```python
from build123d import *

# Parameters (mm, degrees)
SKETCH_1_R      = 5
EXTRUDE_1_DEPTH = 1
SKETCH_3_R      = 3
SKETCH_2_R      = 3.75


with BuildPart() as part:
    # Эскиз1 → Бобышка-Вытянуть1 (new body)
    with BuildSketch(Plane.XY):
        with BuildLine():
            Line((-57.368421028, 25.472814244), (-33.289473642, 43.781399484))
            ThreePointArc((-33.289473642, 43.781399484), (54.999999965, 0), (-33.289473642, -43.781399484))
            Line((-33.289473642, -43.781399484), (-57.368421028, -25.472814244))
            ThreePointArc((-57.368421028, -25.472814244), (-69.999999979, 0), (-57.368421028, 25.472814244))
        make_face()
        with Locations((-22.5, 38.97114317)):
            Circle(SKETCH_1_R, mode=Mode.SUBTRACT)
        with Locations((45, 0)):
            Circle(SKETCH_1_R, mode=Mode.SUBTRACT)
        with Locations((-22.5, -38.97114317)):
            Circle(SKETCH_1_R, mode=Mode.SUBTRACT)
        with BuildLine():
            Line((-45.894736842, 18.375884474), (-13.815789474, 32.157797829))
            ThreePointArc((-13.815789474, 32.157797829), (35, 0), (-13.815789474, -32.157797829))
            Line((-13.815789474, -32.157797829), (-45.894736842, -18.375884474))
            ThreePointArc((-45.894736842, -18.375884474), (-58, 0), (-45.894736842, 18.375884474))
        make_face(mode=Mode.SUBTRACT)
    extrude(amount=EXTRUDE_1_DEPTH)

    # Эскиз3 → Вырез-По сечениям1 section 0
    with BuildSketch(Plane.XY.offset(21)):
        with Locations((0, 45)):
            Circle(SKETCH_3_R)
    # Эскиз2 → Вырез-По сечениям1 section 1
    with BuildSketch(Plane(origin=(0, 0, -24), x_dir=(-1, 0, 0), z_dir=(0, 0, -1))):
        with Locations((0, 45)):
            Circle(SKETCH_2_R)
    loft_1 = loft(mode=Mode.SUBTRACT)

    # Зеркальное отражение1: Вырез-По сечениям1 across plane
    add(loft_1.mirror(Plane.ZX), mode=Mode.SUBTRACT)


solid = part.part
```
The listing builds one solid part. Answer for the finished solid, in the listing's coordinates (mm). A direction names the side the tool comes from. Give positions to 0.01 mm unless a question says otherwise; leave off trailing zeros. Loops run counter-clockwise (first coordinate to the right, second up) from the corner with the lowest first, then second, coordinate; pieces in that order, holes last. Notation, with made-up numbers: M -5.75,2 L 6.25,2 A21 ccw 6.25,19 Z; hole C 8,-22 d8. An arc over 180 degrees is marked long. One line per item, written item: value.
1. Section B-B on x = -22.5 is taken. Determine the outline of the cut face in (y, z).
Found:
outline: M -50.19,0 L -43.97,0 L -43.97,1 L -50.19,1 Z; M -33.97,0 L -28.43,0 L -28.43,1 L -33.97,1 Z; M 28.43,0 L 33.97,0 L 33.97,1 L 28.43,1 Z; M 43.97,0 L 50.19,0 L 50.19,1 L 43.97,1 Z
2. Find the intervals of material crossed by probe 1 along Y at (x, z) = (-22.5, 0.5); probe 2 along Y at (x, z) = (-0.5, 0.5); probe 3 along X at (y, z) = (-39.5, 0.3), in increasing order.
Found:
probe 1: -50.19 to -43.97, -33.97 to -28.43, 28.43 to 33.97, 43.97 to 50.19
probe 2: -55 to -48.3, -41.7 to -35, 35 to 41.7, 48.3 to 55
probe 3: -38.92 to -27.47, -17.53 to 38.27
3. For faces 4 (the face through (-29.631, -25.363, 0.493)), 5 (the face through (-69.997, -0.412, 0.493)), determine the directions among +Z, -Z, +X, -X, +Y, -Y from which every point of the face is accessible in a straight line to the end or side of a thin tool.
Found:
face 4: +Z, -Z
face 5: +Z, -Z, -X
4. For a pull along Y with two mould halves and no side action, classify faces 1 (the face through (-45.16, -34.755, 0.493)), 2 (the face through (-0.435, 48.312, 0.604)), 3 (the face through (35, -11, 1)) as pulls with the +Y half, pulls with the -Y half, needs draft (parallel to the pull), parting line crosses it, or undercut.
Found:
face 1: pulls with the -Y half
face 2: undercut
face 3: needs draft
5. This flat-tipped pin is pushed along its axis until it touches: P1, Ø6, axis at x = 45, y = 0, coming from the +Z side. Where does it stop, or does it pass through?
Found:
P1: through
6. Section D-D on z = 0.5 is taken. Determine the outline of the cut face in (x, y).
Found:
outline: M -57.37,-25.47 L -33.29,-43.78 A55 ccw long -33.29,43.78 L -57.37,25.47 A32 ccw Z; hole M -45.89,-18.38 L -13.82,-32.16 A35 ccw long -13.82,32.16 L -45.89,18.38 A20 ccw Z; hole C -22.5,-38.97 d10; hole C -22.5,38.97 d10; hole C 0,-45 d6.68; hole C 0,45 d6.68; hole C 45,0 d10
7. Section A-A on y = 0 is taken. Determine the outline of the cut face in (x, z).
Found:
outline: M -70,0 L -58,0 L -58,1 L -70,1 Z; M 35,0 L 40,0 L 40,1 L 35,1 Z; M 50,0 L 55,0 L 55,1 L 50,1 Z
8. Section C-C on y = 21.5 is taken. Determine the outline of the cut face in (x, z).
Found:
outline: M -61.7,0 L -38.62,0 L -38.62,1 L -61.7,1 Z; M 27.62,0 L 50.62,0 L 50.62,1 L 27.62,1 Z
